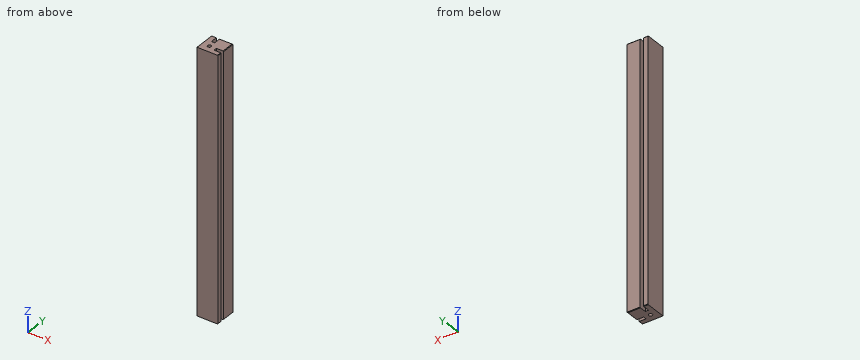
from build123d import *

# Parameters (mm, degrees)
ESQUISSE1_W                      = 16
ESQUISSE1_H                      = 16
BOSS_EXTRU_1_DEPTH               = 200
ESQUISSE2_W                      = 2.5
ESQUISSE2_H                      = 5.5
ESQUISSE2_W_2                    = 5.5
ESQUISSE2_H_2                    = 2.5
ENL_V_MAT_EXTRU_1_DEPTH          = 201.319744409
CHANFREIN1_SIZE                  = 0.4
D_GAGEMENT_M2_51_D               = 2.7
D_GAGEMENT_M2_51_DEPTH           = 14.188838164
D_GAGEMENT_M2_51_TIP             = 0.811161836
D_GAGEMENT_M2_51_ON_FACE_2_D     = 2.7
D_GAGEMENT_M2_51_ON_FACE_2_DEPTH = 14.188838164
D_GAGEMENT_M2_51_ON_FACE_2_TIP   = 0.811161836


with BuildPart() as part:
    # Esquisse1 → Boss.-Extru.1 (new body)
    with BuildSketch(Plane.XY):
        Rectangle(ESQUISSE1_W, ESQUISSE1_H)
    extrude(amount=BOSS_EXTRU_1_DEPTH)

    # Esquisse2 → Enlèv. mat.-Extru.1 (cut, through all)
    with BuildSketch(Plane.XY.offset(200)):
        with Locations((-3.25, 5.25)):
            Rectangle(ESQUISSE2_W, ESQUISSE2_H)
        with Locations((5.25, -3.25)):
            Rectangle(ESQUISSE2_W_2, ESQUISSE2_H_2)
    extrude(amount=-ENL_V_MAT_EXTRU_1_DEPTH, mode=Mode.SUBTRACT)

    # Chanfrein1
    chanfrein1_edges = [part.edges().sort_by_distance(p)[0] for p in [
        (8, 3, 0),
        (-6.25, 8, 0),
        (8, 3, 200),
        (-6.25, 8, 200),
        (8, -6.25, 200),
        (3, 8, 0),
        (8, -6.25, 0),
        (3, 8, 200),
    ]]
    chamfer(chanfrein1_edges, length=CHANFREIN1_SIZE)

    # Dégagement M2.51
    with Locations(Plane(origin=(-2.5, -2.5, 200), x_dir=(1, 0, 0), z_dir=(0, 0, 1))):
        with Locations((0, 0)):
            Hole(D_GAGEMENT_M2_51_D / 2, depth=D_GAGEMENT_M2_51_DEPTH)
            with Locations((0, 0, -(D_GAGEMENT_M2_51_DEPTH + D_GAGEMENT_M2_51_TIP / 2))):  # 118° drill point
                Cone(0, D_GAGEMENT_M2_51_D / 2, D_GAGEMENT_M2_51_TIP, mode=Mode.SUBTRACT)

    # Dégagement M2.51 on face 2
    with Locations(Plane(origin=(-2.5, -2.5, 0), x_dir=(-1, 0, 0), z_dir=(0, 0, -1))):
        with Locations((0, 0)):
            Hole(D_GAGEMENT_M2_51_ON_FACE_2_D / 2, depth=D_GAGEMENT_M2_51_ON_FACE_2_DEPTH)
            with Locations((0, 0, -(D_GAGEMENT_M2_51_ON_FACE_2_DEPTH + D_GAGEMENT_M2_51_ON_FACE_2_TIP / 2))):  # 118° drill point
                Cone(0, D_GAGEMENT_M2_51_ON_FACE_2_D / 2, D_GAGEMENT_M2_51_ON_FACE_2_TIP, mode=Mode.SUBTRACT)


solid = part.part
Design review of the part built by this model. Coordinates are the model's own, in mm. Give positions to 0.01 mm unless a question says otherwise; leave off trailing zeros. Write each loop counter-clockwise with the first axis right and the second up, starting at its lowest first coordinate (ties: lowest second). Pieces come first, ordered by that corner, then holes. Notation, with made-up numbers: M 83,21.25 L 132,21.25 A15 ccw 132,34.25 Z; hole C 62.25,35 d2. An arc over 180 degrees is marked long. Answer as a JSON object with one key per item and string values. Group by question number.
1) For line 1 along X through (y, z) = (3.25, 165.5); line 2 along Y through (x, z) = (-2.5, 194), list the stretches that pass through material, from the lowest coordinate up.
2) We need section B-B (z = 66). Give the boundary of the cut face in (x, y), and give its area (4 significant figures).
3) Clearance check with flat-ended pins moving along their axes: pin 1 Ø2.5 at (x, y) = (-2.5, -2.5) entering from +Z; pin 2 Ø1.2 at (y, z) = (-3, 74) entering from +X. State where each tip first meets the part, or that it passes through.
4) We need section A-A (x = 5.5). Give the boundary of the cut face in (y, z).
Answer key:
{
 "1": {"line 1": "x = -8 to -4.5, -2 to 8", "line 2": "y = -8 to -3.85, -1.15 to 2.5"},
 "2": {"outline": "M -8,-8 L 8,-8 L 8,-4.5 L 2.5,-4.5 L 2.5,-2 L 8,-2 L 8,8 L -2,8 L -2,2.5 L -4.5,2.5 L -4.5,8 L -8,8 Z", "area": "228.5 mm²"},
 "3": {"pin 1": "stops at z = 185.75", "pin 2": "stops at x = 2.5"},
 "4": {"outline": "M -8,0 L -4.5,0 L -4.5,200 L -8,200 Z; M -2,0 L 7.6,0 L 8,0.4 L 8,199.6 L 7.6,200 L -2,200 Z"}
}
